Can you work these out from the model? Positions are in its coordinate system, mm. Face numbers are marked on the shaded views. A direction names the side the tool comes from. Give positions to 0.01 mm unless a question says otherwise; leave off trailing zeros. Write each loop counter-clockwise with the first axis right and the second up, starting at its lowest first coordinate (ties: lowest second). Pieces come first, ordered by that corner, then holes. Notation, with made-up numbers: (-10.75, -30.75) - (27.25, -30.75) arc R17 cw to (27.25, -19.75) - close; hole circle Ø2 at (61, 74.25). An arc over 180 degrees is marked (long way). Return JSON: item names as keys, results as strings. Group by question number.
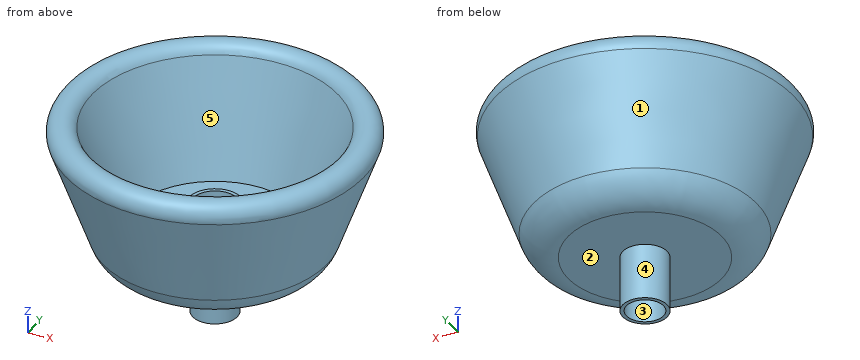
from build123d import *

# Parameters (mm, degrees)
F2_R     = 14
F2_R_2   = 12
F3_DEPTH = 30
F2_R_3   = 10
F4_DEPTH = 30


with BuildPart() as f1:
    # F0 (on Front) → F1 (revolve)
    with BuildSketch(Plane.XZ):
        with BuildLine():
            Line((0, 15), (0, 0))
            Line((0, 0), (41.498962, 0))
            ThreePointArc((41.498962, 0), (52.970491, 3.616959), (60.292815, 13.159597))
            Line((60.292815, 13.159597), (80.229376, 67.934849))
            ThreePointArc((80.229376, 67.934849), (75.746832, 77.547695), (66.133987, 73.065151))
            Line((66.133987, 73.065151), (45, 15))
            Line((45, 15), (0, 15))
        make_face()
    revolve(axis=Axis((0, 0, 7.5), (0, 0, -1)))

    # F2 (on Top) → F3 (join)
    with BuildSketch(Plane.XY):
        Circle(F2_R)
        Circle(F2_R_2, mode=Mode.SUBTRACT)
    extrude(amount=F3_DEPTH)

    # F2 (on Top) → F4 (join)
    with BuildSketch(Plane.XY):
        Circle(F2_R_2)
        Circle(F2_R_3, mode=Mode.SUBTRACT)
    extrude(amount=-F4_DEPTH)


solid = f1.part
1) Will these pins go through, and if not, where does the flat tip stop? pin 1 Ø10 at (x, y) = (4.5, 0.5) entering from -Z; pin 2 Ø3 at (x, z) = (56.5, 21) entering from +Y; pin 3 Ø8.5 at (x, y) = (1, -4.5) entering from +Z.
2) Imagine slicing it at D-D, the plane z = 25. Write out the boundary of the cut face in (x, y), and give its area (3 significant figures).
3) I need wall thicknesses on line 1 along Y through (x, z) = (0, 22.5); line 2 along X through (y, z) = (0, 25.75); line 3 along Z through (x, y) = (17, -4). Which ranges of each line are inside material? Lowest first, please.
4) We'd pull the mould along Y, two halves only. Please class the marked faces 1, 2 and 3: pulls with the +Y half, pulls with the -Y half, needs draft (parallel to the pull), parting line crosses it, or undercut.
5) On a 3-axis mill with a long thin cutter (end or side, diameter ignored), from which of +Z, -Z, +X, -X, +Y, -Y can I reach the whole of each face in a straight line? I mean the marked faces 4 and 5. Say none if no direction works.
6) Imagine slicing it at A-A, the plane x = 0. Write out the boundary of the cut face in (y, z).
7) Imagine slicing it at C-C, the plane z = -5.5. Write out the boundary of the cut face in (x, y), and give its area (3 significant figures).
Resolved:
{
 "1": {"pin 1": "z = 0", "pin 2": "y = 31.25", "pin 3": "z = 15"},
 "2": {"outline": "circle Ø129.2 at (0, 0); circle Ø28 at (0, 0); hole circle Ø97.28 at (0, 0); hole circle Ø24 at (0, 0)", "area": "5,840 mm^2"},
 "3": {"line 1": "-63.69 to -47.73, -14 to -12, 12 to 14, 47.73 to 63.69", "line 2": "-64.88 to -48.91, -14 to -12, 12 to 14, 48.91 to 64.88", "line 3": "0 to 15"},
 "4": {"face 1": "parting line crosses it", "face 2": "needs draft", "face 3": "undercut"},
 "5": {"face 4": "-Z", "face 5": "+Z"},
 "6": {"outline": "(-80.23, 67.93) - (-60.29, 13.16) arc R20 ccw to (-41.5, 0) - (-12, 0) - (-12, -30) - (-10, -30) - (-10, 0) - (10, 0) - (10, -30) - (12, -30) - (12, 0) - (41.5, 0) arc R20 ccw to (60.29, 13.16) - (80.23, 67.93) arc R7.5 ccw to (66.13, 73.07) - (45, 15) - (14, 15) - (14, 30) - (12, 30) - (12, 15) - (-12, 15) - (-12, 30) - (-14, 30) - (-14, 15) - (-45, 15) - (-66.13, 73.07) arc R7.5 ccw to start"},
 "7": {"outline": "circle Ø24 at (0, 0); hole circle Ø20 at (0, 0)", "area": "138 mm^2"}
}
